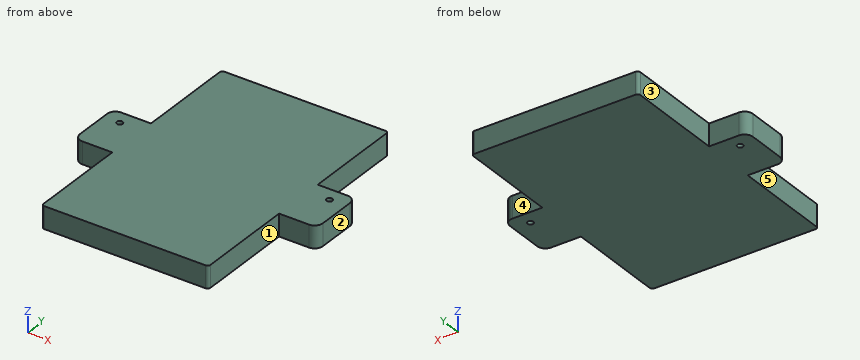
```python
from build123d import *

# Parameters (mm, degrees)
SKETCH_W     = 60.4
SKETCH_H     = 93
PAD_DEPTH    = 8
SKETCH001_W  = 88
SKETCH001_H  = 20
PAD001_DEPTH = 8
SKETCH002_R  = 1.05
POCKET_DEPTH = 264.570679
FILLET_R     = 3
FILLET001_R  = 1


with BuildPart() as part:
    # Sketch → Pad (new body)
    with BuildSketch(Plane.XY):
        Rectangle(SKETCH_W, SKETCH_H)
    extrude(amount=PAD_DEPTH)

    # Sketch001 → Pad001 (join)
    with BuildSketch(Plane.XY):
        Rectangle(SKETCH001_W, SKETCH001_H)
    extrude(amount=PAD001_DEPTH)

    # Sketch002 (on Face10 of Pad001) → Pocket (cut, through all)
    with BuildSketch(Plane.XY.offset(8)):
        with Locations((-38, 5)):
            Circle(SKETCH002_R)
    pocket = extrude(amount=-POCKET_DEPTH, mode=Mode.SUBTRACT)

    # Fillet
    fillet_edges = [part.edges().sort_by_distance(p)[0] for p in [
        (-44, -10, 4),
        (44, -10, 4),
        (44, 10, 4),
        (-44, 10, 4),
    ]]
    fillet(fillet_edges, radius=FILLET_R)

    # Mirrored: Pocket across Sketch002 V_Axis
    add(pocket.mirror(Plane(origin=(0, 0, 8), x_dir=(0, 0, 1), z_dir=(1, 0, 0))), mode=Mode.SUBTRACT)

    # Fillet001
    fillet001_edges = [part.edges().sort_by_distance(p)[0] for p in [
        (-30.2, -46.5, 4),
        (30.2, -46.5, 4),
        (30.2, 46.5, 4),
        (-30.2, 46.5, 4),
    ]]
    fillet(fillet001_edges, radius=FILLET001_R)


solid = part.part
```
Model file for the job. Use its own axes, mm. Face numbers are marked on the shaded views. A direction names the side the tool comes from. Coordinates: 2 decimals unless noted, no trailing zeros. Loops run counter-clockwise (first coordinate to the right, second up) from the corner with the lowest first, then second, coordinate; pieces in that order, holes last. Notation, with made-up numbers: (12, -33) -> (16, -33) arc R21 ccw to (16, -23) -> close; hole circle Ø4 at (-22, -32). An arc over 180 degrees is marked (long way). Answer as a JSON object with one key per item and string values.
Q1. Cut at A-A (y = 5). List the corners of the cut face in (x, z), and give its area (3 significant figures).
Report:
{"outline": "(-44, 0) -> (-39.05, 0) -> (-39.05, 8) -> (-44, 8) -> close; (-36.95, 0) -> (36.95, 0) -> (36.95, 8) -> (-36.95, 8) -> close; (39.05, 0) -> (44, 0) -> (44, 8) -> (39.05, 8) -> close", "area": "670 mm2"}
Q2. Cut at D-D (y = 31.5). List the corners of the cut face in (x, z).
Report:
{"outline": "(-30.2, 0) -> (30.2, 0) -> (30.2, 8) -> (-30.2, 8) -> close"}
Q3. Cut at B-B (x = -38). List the corners of the cut face in (y, z).
Report:
{"outline": "(-10, 0) -> (3.95, 0) -> (3.95, 8) -> (-10, 8) -> close; (6.05, 0) -> (10, 0) -> (10, 8) -> (6.05, 8) -> close"}
Q4. Flat gauge pins, fed straight in: P1, Ø2.5, axis at y = -31.5, z = 3, coming from the -X side; P2, Ø1.7, axis at x = -38, y = 5, coming from the -Z side; P3, Ø4, axis at x = -35.5, z = 5, coming from the -Y side. Where does each tip first touch, or does it go through?
Report:
{"P1": "stops at x = -30.2", "P2": "passes through", "P3": "stops at y = -10"}
Q5. Cut at C-C (z = 5.5). List the corners of the cut face in (x, y), and give its area (3 significant figures).
Report:
{"outline": "(-44, -7) arc R3 ccw to (-41, -10) -> (-30.2, -10) -> (-30.2, -45.5) arc R1 ccw to (-29.2, -46.5) -> (29.2, -46.5) arc R1 ccw to (30.2, -45.5) -> (30.2, -10) -> (41, -10) arc R3 ccw to (44, -7) -> (44, 7) arc R3 ccw to (41, 10) -> (30.2, 10) -> (30.2, 45.5) arc R1 ccw to (29.2, 46.5) -> (-29.2, 46.5) arc R1 ccw to (-30.2, 45.5) -> (-30.2, 10) -> (-41, 10) arc R3 ccw to (-44, 7) -> close; hole circle Ø2.1 at (-38, 5); hole circle Ø2.1 at (38, 5)", "area": "6,150 mm2"}
Q6. Probe probe 1 along Y at (x, z) = (-38, 3); probe 2 along X at (y, z) = (-18, 6.5); probe 3 along Y at (x, z) = (36.5, 3.25). List the from-to ranges inside material, lowest first.
Report:
{"probe 1": "y = -10 to 3.95, 6.05 to 10", "probe 2": "x = -30.2 to 30.2", "probe 3": "y = -10 to 10"}
Q7. 3-axis set-ups, long thin cutter, end or side, ignore diameter. For the marked faces 1, 2, 3, 4 and 5: which of +Z, -Z, +X, -X, +Y, -Y reach the whole face in a straight line?
Report:
{"face 1": "+Z, -Z, +X, -Y", "face 2": "+Z, -Z, +X, +Y, -Y", "face 3": "+Z, -Z, -X, +Y", "face 4": "+Z, -Z, +X, +Y", "face 5": "+Z, -Z, -X, -Y"}
